Build history of the part. All positions in model axes, mm. A direction names the side the tool comes from. Give positions to 0.01 mm unless a question says otherwise; leave off trailing zeros. Order: outer loops, then holes, each group sorted by start corner. A loop starts at its lowest first (then second) coordinate and runs counter-clockwise, first axis right, second up. Notation, with made-up numbers: M 89,15 L 121,15 A7 cw 121,28 Z; hole C -12.5,30.25 d7. An arc over 180 degrees is marked long. One line per item, written item: value. Start each with the question number.
Autodesk Inventor part; units mm, degrees
ref_plane "YZ Plane" through (0, 0, 0) normal (1, 0, 0) x (0, 1, 0)
ref_plane "XZ Plane" through (0, 0, 0) normal (0, 1, 0) x (-1, 0, 0)
ref_plane "XY Plane" through (0, 0, 0) normal (0, 0, 1) x (1, 0, 0)
sketch "Sketch1" plane through (0, 0, 0) normal (0, 0, 1) x (1, 0, 0)
  line L0 (0, 0) -> (0, 53.5)
  line L1 (0, 53.5) -> (30, 53.5)
  line L2 (30, 53.5) -> (30, 43.5)
  line L3 (30, 43.5) -> (10, 23.5)
  line L4 (10, 23.5) -> (10, 0)
  line L5 (-6, 0) -> (36, 0)
  line L6 (0, 0) -> (0, -53.5)
  line L7 (0, -53.5) -> (30, -53.5)
  line L8 (30, -53.5) -> (30, -43.5)
  line L9 (30, -43.5) -> (10, -23.5)
  line L10 (10, -23.5) -> (10, 0)
  dimension "d0" = 53.5
  dimension "d1" = 10
  dimension "d2" = 10
  dimension "d3" = 135
  dimension "d4" = 30
extrude "Extrusion1" add sketch "Sketch1" along normal blind 6
sketch "Sketch2" plane through (0, 0, 0) normal (0, 0, 1) x (1, 0, 0)
  line L0 (0, -53.5) -> (30, -53.5)
  line L1 (0, 53.5) -> (0, -53.5)
  line L2 (30, 53.5) -> (0, 53.5)
  line L3 (30, 53.5) -> (0, 53.5)
  line L4 (30, 53.5) -> (30, 59.5)
  line L5 (30, 59.5) -> (-6, 59.5)
  line L6 (-6, 59.5) -> (-6, -59.5)
  line L7 (-6, -59.5) -> (30, -59.5)
  line L8 (30, -59.5) -> (30, -53.5)
  point P0 (0, 0)
  dimension "d7" = 6
  dimension "d8" = 6
  dimension "d9" = 6
extrude "Extrusion2" add sketch "Sketch2" along normal blind 31
mirror "Mirror1" about plane through (12, 0, 31) normal (0, 0, 1) of "Extrusion1", "Extrusion2"
sketch "Sketch4" plane through (0, 0, 62) normal (0, 0, 1) x (1, 0, 0)
  line L0 (-6, 59.5) -> (-6, -59.5) construction
  line L1 (30, 59.5) -> (-6, 59.5) construction
  line L2 (-6, 59.5) -> (-31, 59.5)
  line L3 (-31, 59.5) -> (-31, 33.5)
  line L4 (-31, 33.5) -> (-6, 33.5)
  line L5 (-6, 59.5) -> (-6, -59.5)
  line L6 (-6, 59.5) -> (-6, 33.5)
  line L7 (-18, 22.2914) -> (-18, 69.8308) construction
  line L8 (-26.7913, 46.5) -> (-0.8939, 46.5) construction
  circle A0 centre (-18, 46.5) radius 7.5 construction
  circle A1 centre (-25.5, 46.5) radius 1.25
  circle A2 centre (-14.25, 40.0048) radius 1.25
  circle A3 centre (-14.25, 52.9952) radius 1.25
  point P0 (0, 0)
  dimension "d39" = 15
  dimension "d26" = 25
  dimension "d27" = 26
  dimension "d30" = 12
  dimension "d38" = 13
  dimension "d40" = 2.5
  dimension "d43" = 360
extrude "Extrusion3" add sketch "Sketch4" against normal blind 6
chamfer "Chamfer1" distance 7.5 angle 45 2 edges at (-31, 33.5, 59) (-31, 59.5, 59)
chamfer "Chamfer2" distance 12.5 angle 45 1 edges at (-6, 33.5, 59)
chamfer "Chamfer3" distance 3 angle 45 1 edges at (-6, 46.5, 56)
ref_plane "Work Plane1" through (0, 0, 62) normal (-1, 0, 0) x (0, 1, 0)
equation "\"d0\" = 0.5 * width"
equation "\"d1\" = border"
equation "\"d2\" = border"
equation "\"d5\" = wall_thickness"
equation "\"d7\" = wall_thickness"
equation "\"d8\" = wall_thickness"
equation "\"d9\" = wall_thickness"
equation "\"d10\" = wall_thickness + 0.5 * depth"
equation "\"d38\" = 0.5 * d27"
equation "\"d33\" = wall_thickness"
equation "\"width\" = 107"
equation "\"depth\" = 50"
equation "\"border\" = 10"
equation "\"wall_thickness\" = 6"
properties part number "_3DPrint"
1) Slice it at A-A (y = 46.5). List the corners of the cut face in (x, z).
2) Slice it at D-D (y = -36.5). List the corners of the cut face in (x, z), plus the area to 3 significant figures.
3) Tool access for faces 4 (the flat face through (-21, 33.5, 59)), 5 (the flat face through (8, 1, 6)), 6 (the flat face through (-18, 46, 56)), 7 (the flat face through (19.9, -33.4, 59)): list every direction of +Z, -Z, +X, -X, +Y, -Y with a clear straight run to the whole face (end or side of a thin tool).
4) Drill centre lines: line 1 (Z direction, x = 1, y = -28); line 2 (Y direction, x = -14, z = 58); line 3 (Y direction, x = 18.5, z = 15.5). Where is each one in solid material? Low to high.
5) Slice it at C-C (x = 5). List the corners of the cut face in (y, z).
6) Drop flat-ended pins along their axis: P1, Ø12, axis at x = 17, y = -47, coming from the -Z side; P2, Ø11, axis at x = -18.5, y = 49.5, coming from the -Z side; P3, Ø1.5, axis at y = 11, z = 47, coming from the +X side; P4, Ø6.5, axis at y = 1, z = 3.5, coming from the +X side. Give the stop position or say it passes through.
7) Pull direction Z, two halves, no side cores. Call faces 1 (the flat face through (-27, 37, 59)), 2 (the flat face through (8, 1, 0)), 3 (the flat face through (9, 1, 56)): pulls with the +Z half, pulls with the -Z half, needs draft (parallel to the pull), parting line crosses it, or undercut.
8) Slice it at B-B (x = -14.25). List the corners of the cut face in (y, z).
Results list:
1. outline: M -31,56 L -26.75,56 L -26.75,62 L -31,62 Z; M -24.25,56 L -9,56 L -6,53 L -6,0 L 30,0 L 30,6 L 0,6 L 0,56 L 30,56 L 30,62 L -24.25,62 Z
2. outline: M -6,0 L 23,0 L 23,6 L 0,6 L 0,56 L 23,56 L 23,62 L -6,62 Z
2. area: 648 mm²
3. face 4: +Z, -Z, -X, -Y
3. face 5: +X
3. face 6: -Z, -X, +Y, -Y
3. face 7: +Z, -Z, +X
4. line 1: z = 0 to 6, 56 to 62
4. line 2: y = 29 to 38.78, 41.23 to 51.77, 54.22 to 59.5
4. line 3: y = -59.5 to -53.5, 53.5 to 59.5
5. outline: M -59.5,0 L 59.5,0 L 59.5,62 L -59.5,62 Z; hole M -53.5,6 L 53.5,6 L 53.5,56 L -53.5,56 Z
6. P1: stops at z = 0
6. P2: stops at z = 56
6. P3: stops at x = 0
6. P4: stops at x = 10
7. face 1: needs draft
7. face 2: pulls with the -Z half
7. face 3: undercut
8. outline: M 29.25,56 L 38.75,56 L 38.75,62 L 29.25,62 Z; M 41.25,56 L 51.75,56 L 51.75,62 L 41.25,62 Z; M 54.25,56 L 59.5,56 L 59.5,62 L 54.25,62 Z
